Geometry: see drawing. Coordinates: mm, zero at the bounding-box minimum. A direction names the side the tool comes from. Round coordinates to 2 decimals unless told otherwise and drop trailing zeros. Write each loop counter-clockwise with the first axis right and the second up, starting at its lowest first coordinate (ties: lowest second). Pieces come first, ordered by that corner, then holes.
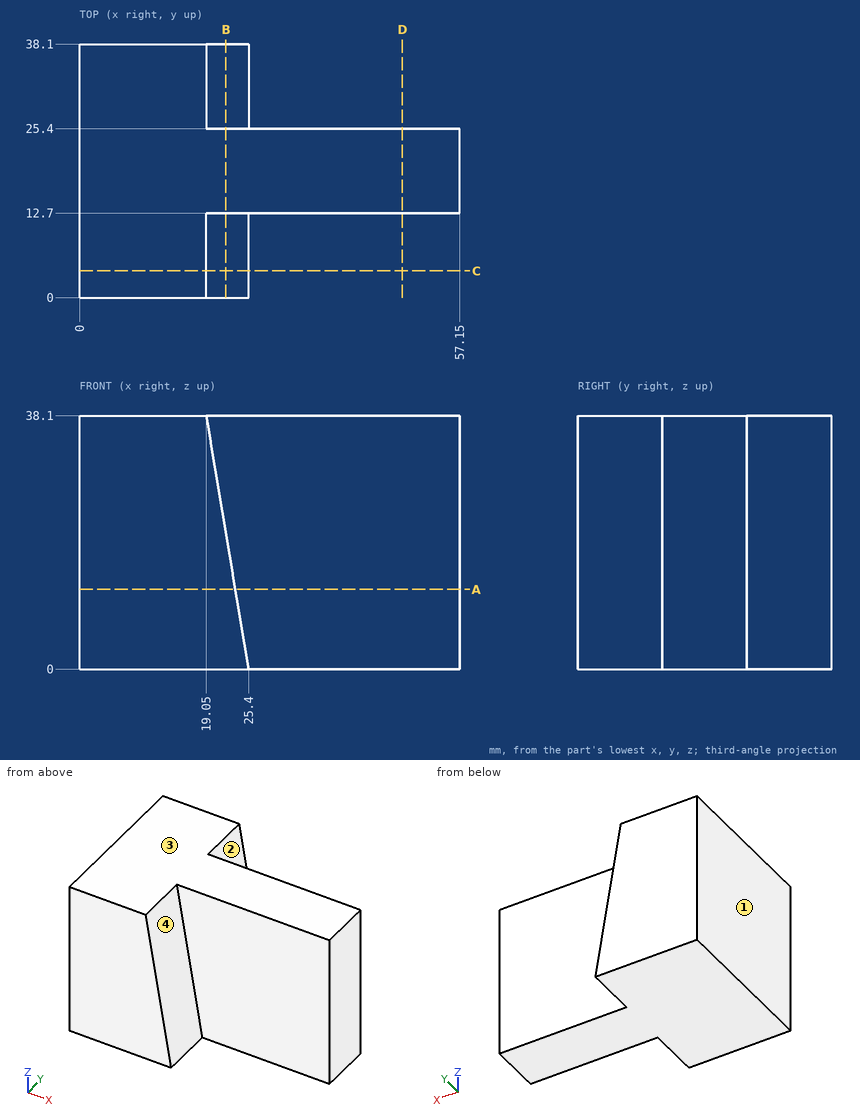
1) Contact query for flat-ended pins moving along their axis: P1, Ø1, axis at y = 20.5, z = 30, coming from the -X side; P2, Ø10, axis at x = 48, z = 12.5, coming from the +Y side; P3, Ø6, axis at y = 7.5, z = 24.5, coming from the +X side. Output: stop coordinate, or through.
Taken from the geometry:
P1: stops at x = 0
P2: stops at y = 25.4
P3: stops at x = 21.82
2) Section query A-A on z = 12. Return the cut outline in (x, y).
Taken from the geometry:
outline: (0, 0) - (23.4, 0) - (23.4, 12.7) - (57.15, 12.7) - (57.15, 25.4) - (23.4, 25.4) - (23.4, 38.1) - (0, 38.1) - close
3) Section query C-C on y = 4. Return the cut outline in (x, z).
Taken from the geometry:
outline: (0, 0) - (25.4, 0) - (19.05, 38.1) - (0, 38.1) - close
4) Reachability of the marked faces 1, 2, 3 and 4 from +Z, -Z, +X, -X, +Y, -Y: full face, straight path, thin tool, end or side. Return the list, or none.
Taken from the geometry:
face 1: +Z, -Z, -X, +Y, -Y
face 2: +Z, +X, +Y
face 3: +Z, +X, -X, +Y, -Y
face 4: +Z, +X, -Y
5) Section query B-B on x = 22. Return the cut outline in (y, z).
Taken from the geometry:
outline: (0, 0) - (38.1, 0) - (38.1, 20.4) - (25.4, 20.4) - (25.4, 38.1) - (12.7, 38.1) - (12.7, 20.4) - (0, 20.4) - close
6) Section query D-D on x = 48.5. Return the cut outline in (y, z).
Taken from the geometry:
outline: (12.7, 0) - (25.4, 0) - (25.4, 38.1) - (12.7, 38.1) - close
7) Material intervals for line 1 (Y direction, x = 38.5, z = 33); line 2 (X direction, y = 36.5, z = 10); line 3 (X direction, y = 25.5, z = 28), sorted ascending.
Taken from the geometry:
line 1: y = 12.7 to 25.4
line 2: x = 0 to 23.73
line 3: x = 0 to 20.73
